Input: part model. Units: mm. Frame: model coordinates. A direction names the side the tool comes from. Round coordinates to 2 decimals unless told otherwise and drop trailing zeros. Loops run counter-clockwise (first coordinate to the right, second up) from the corner with the lowest first, then second, coordinate; pieces in that order, holes last. Notation, with made-up numbers: (1.5, -17) -> (18.5, -17) arc R31 cw to (18.5, 16) -> close; hole circle Ø6 at (-21, 18.25). An arc over 180 degrees is marked (long way). Answer as a JSON object with one key per item and string values. Group by question number.
Item 1: Draft query along Y for faces 6 (the cylindrical face through (3.62, 3.71, 1.96)), 7 (the cylindrical face through (-3.07, 1.87, 1.59)), 8 (the cylindrical face through (-3.07, 1.87, 5.35)), 9 (the flat face through (3.85, 2.7, 1)). Return one class per face: released by +Y, released by -Y, zero draft, split by the parting line, or undercut.
Item 2: Pin query (flat end, axial travel): pin 1 (1 mm diameter, centred on x = -3, z = 0, fed in from -Y); pin 2 (1.2 mm diameter, centred on y = 2, z = 3.5, fed in from +X); pin 3 (0.7 mm diameter, centred on y = 1.5, z = 1.5, fed in from -X). Return the tip coordinate at first contact, or that it passes through.
Item 3: Set-up query: faces 1 (the flat face through (-3.697, 1.178, 3.9)), 2 (the flat face through (0, 2, 5.4)), 3 (the flat face through (3.696, 0.807, -1.4)), 4 (the flat face through (-0.3, 3.7, 6.4)), 5 (the flat face through (-3.45, 2, -2)). Return all of +Z, -Z, +X, -X, +Y, -Y with unobstructed straight access to the full face (end or side cutting, diameter ignored); none if empty.
Item 4: Material intervals for line 1 (Y direction, x = -1, z = 1.5); line 2 (X direction, y = 2.9, z = 1), sorted ascending. Write a range as [from, to].
Item 5: Section query A-A on z = 4.5. Count the separate pieces of the cut face and the enclosed holes in it, and give its area (3 significant figures).
Item 6: Section query D-D on x = 0.5. Return loops of the section in (y, z), and give its area (3 significant figures).
Item 7: Section query B-B on z = 2.5. Return loops of the section in (x, y), and give its area (3 significant figures).
from build123d import *

# Parameters (mm, degrees)
BODY_START       = 6.4
BODY_DEPTH       = 9
SKETCH2_W        = 2.5
SKETCH2_H        = 2
SKETCH2_W_2      = 7.7
SKETCH2_H_2      = 3.5
BODYCUT_DEPTH    = 2.75
FOOT1_DEPTH      = 0.6
FOOT2_DEPTH      = 0.6
CORE1_DEPTH      = 2.3
CORE2_DEPTH      = 4.5
SKETCH9_R        = 0.4
LOCATEPINS_DEPTH = 0.5


with BuildPart() as part:
    # Sketch1 → Body (new body)
    with BuildSketch(Plane.XY.offset(BODY_START)):
        with BuildLine():
            ThreePointArc((3.6125, 1.975), (3.788241153, 2.235632313), (3.85, 2.543853013))
            Line((3.85, 2.543853013), (3.85, 3.15))
            ThreePointArc((3.85, 3.15), (3.615685425, 3.715685425), (3.05, 3.95))
            Line((3.05, 3.95), (-3.05, 3.95))
            ThreePointArc((-3.05, 3.95), (-3.615685425, 3.715685425), (-3.85, 3.15))
            Line((-3.85, 3.15), (-3.85, 2.543853013))
            ThreePointArc((-3.85, 2.543853013), (-3.788241153, 2.235632313), (-3.6125, 1.975))
            ThreePointArc((-3.6125, 1.975), (-3.436758847, 1.714367687), (-3.375, 1.406146987))
            Line((-3.375, 1.406146987), (-3.375, 0.8))
            ThreePointArc((-3.375, 0.8), (-3.140685425, 0.234314575), (-2.575, 0))
            Line((-2.575, 0), (2.575, 0))
            ThreePointArc((2.575, 0), (3.140685425, 0.234314575), (3.375, 0.8))
            Line((3.375, 0.8), (3.375, 1.406146987))
            ThreePointArc((3.375, 1.406146987), (3.436758847, 1.714367687), (3.6125, 1.975))
        make_face()
        with BuildLine():
            ThreePointArc((3.33125, 2.259426506), (3.419120577, 2.389742663), (3.45, 2.543853013))
            Line((3.45, 2.543853013), (3.45, 3.15))
            ThreePointArc((3.45, 3.15), (3.332842712, 3.432842712), (3.05, 3.55))
            Line((3.05, 3.55), (-3.05, 3.55))
            ThreePointArc((-3.05, 3.55), (-3.332842712, 3.432842712), (-3.45, 3.15))
            Line((-3.45, 3.15), (-3.45, 2.543853013))
            ThreePointArc((-3.45, 2.543853013), (-3.419120577, 2.389742663), (-3.33125, 2.259426506))
            ThreePointArc((-3.33125, 2.259426506), (-3.06763827, 1.868478038), (-2.975, 1.406146987))
            Line((-2.975, 1.406146987), (-2.975, 0.8))
            ThreePointArc((-2.975, 0.8), (-2.857842712, 0.517157288), (-2.575, 0.4))
            Line((-2.575, 0.4), (2.575, 0.4))
            ThreePointArc((2.575, 0.4), (2.857842712, 0.517157288), (2.975, 0.8))
            Line((2.975, 0.8), (2.975, 1.406146987))
            ThreePointArc((2.975, 1.406146987), (3.06763827, 1.868478038), (3.33125, 2.259426506))
        make_face(mode=Mode.SUBTRACT)
    extrude(amount=-BODY_DEPTH)

    # Sketch2 → BodyCut (cut)
    with BuildSketch(Plane.XZ):
        with Locations((2.6, 3.27)):
            Rectangle(SKETCH2_W, SKETCH2_H)
        with Locations((0, -0.85)):
            Rectangle(SKETCH2_W_2, SKETCH2_H_2)
        with Locations((-2.6, 3.27)):
            Rectangle(SKETCH2_W, SKETCH2_H)
    extrude(amount=-BODYCUT_DEPTH, mode=Mode.SUBTRACT)

    # Sketch3 → Foot1 (add, symmetric)
    with BuildSketch(Plane.XY.offset(-2)):
        with BuildLine():
            Line((-3.45, 2.75), (-3.45, 0.8))
            ThreePointArc((-3.45, 0.8), (-3.684314575, 0.234314575), (-4.25, 0))
            Line((-4.25, 0), (-4.95, 0))
            Line((-4.95, 0), (-4.95, 0.4))
            Line((-4.95, 0.4), (-4.25, 0.4))
            ThreePointArc((-4.25, 0.4), (-3.967157288, 0.517157288), (-3.85, 0.8))
            Line((-3.85, 0.8), (-3.85, 2.75))
            Line((-3.85, 2.75), (-3.45, 2.75))
        make_face()
    foot1 = extrude(amount=FOOT1_DEPTH, both=True)

    # Sketch4 → Foot2 (add, symmetric)
    with BuildSketch(Plane.XY.offset(3.3)):
        with BuildLine():
            Line((-3.45, 2.75), (-3.45, 0.8))
            ThreePointArc((-3.45, 0.8), (-3.684314575, 0.234314575), (-4.25, 0))
            Line((-4.25, 0), (-4.95, 0))
            Line((-4.95, 0), (-4.95, 0.4))
            Line((-4.95, 0.4), (-4.25, 0.4))
            ThreePointArc((-4.25, 0.4), (-3.967157288, 0.517157288), (-3.85, 0.8))
            Line((-3.85, 0.8), (-3.85, 2.75))
            Line((-3.85, 2.75), (-3.45, 2.75))
        make_face()
    foot2 = extrude(amount=FOOT2_DEPTH, both=True)

    # Mirror1: Foot1, Foot2 across plane
    add(foot1.mirror(Plane(origin=(0, 0, 0), x_dir=(0, 0, 1), z_dir=(1, 0, 0))))
    add(foot2.mirror(Plane(origin=(0, 0, 0), x_dir=(0, 0, 1), z_dir=(1, 0, 0))))

    # Sketch6 → Core1 (add)
    with BuildSketch(Plane(origin=(0, 0, 0.9), x_dir=(-1, 0, 0), z_dir=(0, 0, -1))):
        with BuildLine():
            Line((3.45, 3.15), (3.45, 2.75))
            Line((3.45, 2.75), (3.85, 2.75))
            Line((3.85, 2.75), (3.85, 2.543853013))
            ThreePointArc((3.85, 2.543853013), (3.788241153, 2.235632313), (3.6125, 1.975))
            ThreePointArc((3.6125, 1.975), (3.436758847, 1.714367687), (3.375, 1.406146987))
            Line((3.375, 1.406146987), (3.375, 0.8))
            ThreePointArc((3.375, 0.8), (3.140685425, 0.234314575), (2.575, 0))
            Line((2.575, 0), (-2.575, 0))
            ThreePointArc((-2.575, 0), (-3.140685425, 0.234314575), (-3.375, 0.8))
            Line((-3.375, 0.8), (-3.375, 1.406146987))
            ThreePointArc((-3.375, 1.406146987), (-3.436758847, 1.714367687), (-3.6125, 1.975))
            ThreePointArc((-3.6125, 1.975), (-3.788241153, 2.235632313), (-3.85, 2.543853013))
            Line((-3.85, 2.543853013), (-3.85, 2.75))
            Line((-3.85, 2.75), (-3.45, 2.75))
            Line((-3.45, 2.75), (-3.45, 3.15))
            ThreePointArc((-3.45, 3.15), (-3.332842712, 3.432842712), (-3.05, 3.55))
            Line((-3.05, 3.55), (3.05, 3.55))
            ThreePointArc((3.05, 3.55), (3.332842712, 3.432842712), (3.45, 3.15))
        make_face()
    extrude(amount=CORE1_DEPTH)

    # Sketch7 → Core2 (add)
    with BuildSketch(Plane.XY.offset(0.9)):
        Polygon((-2.3, 2.5), (2.3, 2.5), (2.3, 1.6), (1.75, 0.9), (-1.75, 0.9), (-2.3, 1.6), align=None)
    extrude(amount=CORE2_DEPTH)

    # Sketch9 → LocatePins (add)
    with BuildSketch(Plane.XZ):
        with Locations(Location((-1.75, 0, 0), (0, 0, 270))):
            Circle(SKETCH9_R)
        with Locations(Location((1.75, 0, 0), (0, 0, 90))):
            Circle(SKETCH9_R)
    extrude(amount=LOCATEPINS_DEPTH)


solid = part.part
Solved:
{
 "1": {"face 6": "released by +Y", "face 7": "undercut", "face 8": "undercut", "face 9": "zero draft"},
 "2": {"pin 1": "y = 0", "pin 2": "x = 3.85", "pin 3": "x = -3.51"},
 "3": {"face 1": "-X, -Y", "face 2": "+Z", "face 3": "+X, -Y", "face 4": "+Z, +X, -X, +Y, -Y", "face 5": "-Z, -Y"},
 "4": {"line 1": "[0, 0.4], [0.9, 2.5], [3.55, 3.95]", "line 2": "[-3.85, -3.45], [3.45, 3.85]"},
 "5": {"separate pieces": "2", "enclosed holes": "1", "area": "15.0 mm²"},
 "6": {"outline": "(0, -1.4) -> (3.55, -1.4) -> (3.55, -2.6) -> (3.95, -2.6) -> (3.95, 6.4) -> (3.55, 6.4) -> (3.55, 0.9) -> (2.5, 0.9) -> (2.5, 5.4) -> (0.9, 5.4) -> (0.9, 0.9) -> (0.4, 0.9) -> (0.4, 6.4) -> (0, 6.4) -> close", "area": "21.2 mm²"},
 "7": {"outline": "(-3.85, 2.75) -> (-3.45, 2.75) -> (-3.45, 3.15) arc R0.4 cw to (-3.05, 3.55) -> (3.05, 3.55) arc R0.4 cw to (3.45, 3.15) -> (3.45, 2.75) -> (3.85, 2.75) -> (3.85, 3.15) arc R0.8 ccw to (3.05, 3.95) -> (-3.05, 3.95) arc R0.8 ccw to (-3.85, 3.15) -> close; (-2.3, 1.6) -> (-1.75, 0.9) -> (1.75, 0.9) -> (2.3, 1.6) -> (2.3, 2.5) -> (-2.3, 2.5) -> close; (-1.35, 0) -> (1.35, 0) -> (1.35, 0.4) -> (-1.35, 0.4) -> close", "area": "11.6 mm²"}
}
